Autodesk Inventor part; units mm, degrees
ref_plane "YZ Plane" through (0, 0, 0) normal (1, 0, 0) x (0, 1, 0)
ref_plane "XZ Plane" through (0, 0, 0) normal (0, 1, 0) x (-1, 0, 0)
ref_plane "XY Plane" through (0, 0, 0) normal (0, 0, 1) x (1, 0, 0)
sketch "Skizze1" plane through (0, 0, 0) normal (0, 0, 1) x (1, 0, 0)
  circle A0 centre (0, 0) radius 3.5
  dimension "d0" = 7
extrude "Extrusion1" add sketch "Skizze1" along normal blind 16.5
sketch "Skizze2" plane through (0, 0, 16.5) normal (0, 0, 1) x (1, 0, 0)
  circle A0 centre (0, 0) radius 1
  dimension "d3" = 2
extrude "Extrusion2" add sketch "Skizze2" along normal blind 7.75
fillet "Rundung1" radius 0.5 2 edges at (-3.5, 0, 16.5) (-3.5, 0, 0)
properties part number "P_Motor"
Check sheet for the modelled part. Datum: model origin and axes. Units: mm. A direction names the side the tool comes from. Round coordinates to 2 decimals unless told otherwise and drop trailing zeros. Order: outer loops, then holes, each group sorted by start corner. A loop starts at its lowest first (then second) coordinate and runs counter-clockwise, first axis right, second up. Notation, with made-up numbers: M 85,77.25 L 92,77.25 A24 ccw 92,115.25 Z; hole C 47,-28.5 d1. An arc over 180 degrees is marked long. One line per item, written item: value. Start each with the question number.
1. Scan lines: line 1 along Z through (x, y) = (-0.25, -2); line 2 along Y through (x, z) = (-2.75, 9.25); line 3 along Y through (x, z) = (2, 11.5). Record each from-to range of solid material in increasing order.
2. Gauge pin test, flat ends, axial feed: P1, Ø1, axis at x = -2.5, y = 2, coming from the +Z side; P2, Ø2, axis at y = 2.5, z = 21, coming from the +X side; P3, Ø1, axis at x = -1.5, z = 13.5, coming from the -Y side; P4, Ø4, axis at x = -2.5, z = 16, coming from the +Y side. Record the tip position at first contact, or that the pin passes through.
3. Access from +Z, -Z, +X, -X, +Y, -Y to the whole of each face (thin tool, end or side, straight path). Record for faces 1 (the flat face through (0, 0, 24.25)), 2 (the cylindrical face through (0, 1, 20)).
4. Section check C-C on z = 5.5. Enter the section's corners in (x, y), and give its area (3 significant figures).
5. Section check A-A on y = 0. Enter the section's corners in (x, z).
6. Section check D-D on z = 18.25. Enter the section's corners in (x, y).
Results found:
1. line 1: 0 to 16.5
1. line 2: -2.17 to 2.17
1. line 3: -2.87 to 2.87
2. P1: z = 16.5
2. P2: through
2. P3: y = -3.35
2. P4: y = 3.46
3. face 1: +Z, +X, -X, +Y, -Y
3. face 2: +Z
4. outline: C 0,0 d7
4. area: 38.5 mm^2
5. outline: M -3.5,0.5 A0.5 ccw -3,0 L 3,0 A0.5 ccw 3.5,0.5 L 3.5,16 A0.5 ccw 3,16.5 L 1,16.5 L 1,24.25 L -1,24.25 L -1,16.5 L -3,16.5 A0.5 ccw -3.5,16 Z
6. outline: C 0,0 d2
